```python
from build123d import *

# Parameters (mm, degrees)
EXTRUDE_THIN1_DEPTH     = 190.5
EXTRUDE_THIN2_DEPTH     = 241.3
CUT_EXTRUDE3_DEPTH      = 311.192787835
CUT_EXTRUDE3_DEPTH_BACK = 311.192787835
SKETCH5_R               = 4.7625


# Read off the part's stored shape, not the designer's step: Extrude-Thin2
with BuildPart() as part:
    # Sketch1 → Extrude-Thin1 (new, symmetric)
    with BuildSketch(Plane.XY):
        Polygon((38.1, 0), (0, 0), (0, 38.1), (3.175, 38.1), (3.175, 3.175), (38.1, 3.175), align=None)
    extrude(amount=EXTRUDE_THIN1_DEPTH, both=True)

    # Extrude-Thin2 outline → Extrude-Thin2 (add)
    with BuildSketch(Plane.ZY):
        Polygon((190.5, 3.175), (190.5, 6.35), (155.575, 6.35), (155.575, 41.275), (152.4, 41.275), (152.4, 3.175), align=None)
        Polygon((-155.575, 6.35), (-190.5, 6.35), (-190.5, 3.175), (-152.4, 3.175), (-152.4, 41.275), (-155.575, 41.275), align=None)
    extrude(amount=EXTRUDE_THIN2_DEPTH)

    # Sketch5 → Cut-Extrude3 (cut, two sides: drawn at the far end of the back side and taken through both)
    with BuildSketch(Plane.XY.offset(-CUT_EXTRUDE3_DEPTH_BACK)):
        with Locations((-228.6, 28.575)):
            Circle(SKETCH5_R)
        with Locations((-38.1, 28.575)):
            Circle(SKETCH5_R)
    extrude(amount=CUT_EXTRUDE3_DEPTH + CUT_EXTRUDE3_DEPTH_BACK, mode=Mode.SUBTRACT)


solid = part.part
```
Can you work these out from the model? Positions are in its coordinate system, mm. A direction names the side the tool comes from. Round coordinates to 2 decimals unless told otherwise and drop trailing zeros. Loops run counter-clockwise (first coordinate to the right, second up) from the corner with the lowest first, then second, coordinate; pieces in that order, holes last. Notation, with made-up numbers: M 56.25,45 L 92.25,45 A19 ccw 92.25,71 Z; hole C 24.25,-17 d5. An arc over 180 degrees is marked long. Write item = value, one per line. Start each with the question number.
(1) Suppose I cut it at B-B on x = -38.1. Give the number of separate pieces and of enclosed holes in the cut face, plus the area to 3 significant figures.
(2) If we mould it in two halves opening along Y, with no side actions, what happens to faces 1 (the face through (20, 3.175, 3)), 2 (the face through (-224.2, 26.75, -154.01)), 3 (the face through (-80, 6, 190.5))? For each: released by +Y, released by -Y, zero draft, split by the parting line, or undercut.
(3) Which directions (+Z, -Z, +X, -X, +Y, -Y) give clear straight access to the entire face, cutting with the end or side of a thin tool? Please do faces 4 (the face through (-119, 24, 155.575)), 5 (the face through (-119, 6.35, -173)), 6 (the face through (-119, 3.175, 171)), 7 (the face through (3.175, 21, 3)), 8 (the face through (-119, 22, -152.4)).
(4) Suppose I cut it at C-C on z = 139. Write out the boundary of the cut face in (x, y) (3 decimals).
(5) I need wall thicknesses on line 1 along Y through (x, z) = (-38.1, 154.9) (1 decimal); line 2 along Z through (x, y) = (-161, 15) (3 decimals); line 3 along Y through (x, z) = (-228, -154) (3 decimals). Which ranges of each line are inside material? Lowest first, please.
(6) Suppose I cut it at D-D on x = 18. Write out the boundary of the cut face in (y, z) (3 decimals).
(7) Suppose I cut it at A-A on x = -72. Write out the boundary of the cut face in (y, z) (3 decimals).
(8) I'm going to push flat-ended pins straight in: P1, Ø1, axis at x = -173, y = 28, coming from the +Z side (3 decimals); P2, Ø8.5, axis at x = -228.6, y = 28.575, coming from the -Z side; P3, Ø17.5, axis at x = -74.5, y = 19, coming from the -Z side (3 decimals); P4, Ø2.5, axis at y = 39.5, z = 153.5, coming from the +X side. Where does each tip first touch, or does it pass through?
Answer block:
q1.separate_pieces = 4
q1.enclosed_holes = 0
q1.area = 403 mm²
q2.face_1 = released by +Y
q2.face_2 = undercut
q2.face_3 = zero draft
q3.face_4 = +Z, -X, +Y
q3.face_5 = -Z, -X, +Y
q3.face_6 = +Z, -Z, -X, -Y
q3.face_7 = +Z, -Z, +X, +Y
q3.face_8 = -X, +Y, -Y
q4.outline = M 0,0 L 38.1,0 L 38.1,3.175 L 3.175,3.175 L 3.175,38.1 L 0,38.1 Z
q5.line_1 = 3.2 to 23.8, 33.3 to 41.3
q5.line_2 = -155.575 to -152.4, 152.4 to 155.575
q5.line_3 = 3.175 to 23.85, 33.3 to 41.275
q6.outline = M 0,-190.5 L 3.175,-190.5 L 3.175,190.5 L 0,190.5 Z
q7.outline = M 3.175,-190.5 L 6.35,-190.5 L 6.35,-155.575 L 41.275,-155.575 L 41.275,-152.4 L 3.175,-152.4 Z; M 3.175,152.4 L 41.275,152.4 L 41.275,155.575 L 6.35,155.575 L 6.35,190.5 L 3.175,190.5 Z
q8.P1 = 155.575
q8.P2 = through
q8.P3 = -155.575
q8.P4 = 0
